Check sheet for the drawn part. Datum: minimum x, y, z corner. Units: mm. A direction names the side the tool comes from. Coordinates: 2 decimals unless noted, no trailing zeros. Loops run counter-clockwise (first coordinate to the right, second up) from the corner with the lowest first, then second, coordinate; pieces in that order, holes last.
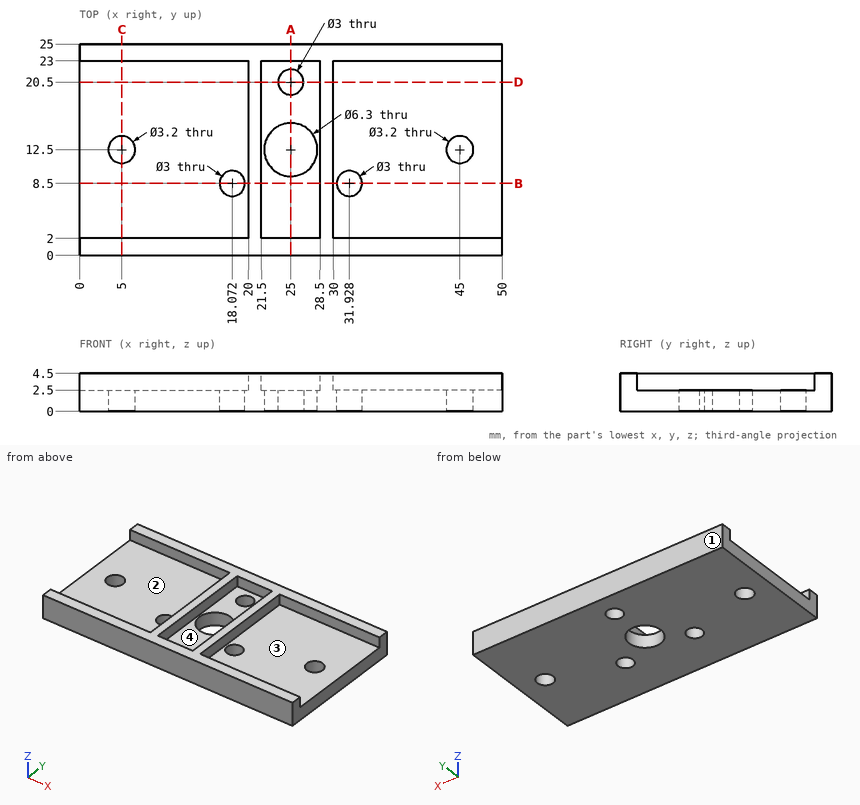
1) Section check C-C on x = 5. Enter the section's corners in (y, z), plus the area to 3 significant figures.
Answer sheet:
outline: (0, 0) - (10.9, 0) - (10.9, 2.5) - (2, 2.5) - (2, 4.5) - (0, 4.5) - close; (14.1, 0) - (25, 0) - (25, 4.5) - (23, 4.5) - (23, 2.5) - (14.1, 2.5) - close
area: 62.5 mm2
2) Mould release check, pull along X, two halves, no side actions. Record for the marked faces 3 and 4: +X half, -X half, draft (parallel to the pull), parting line (faces both ways), or undercut.
Answer sheet:
face 3: draft
face 4: undercut
3) Section check D-D on y = 20.5. Enter the section's corners in (x, z), plus the area to 4 significant figures.
Answer sheet:
outline: (0, 0) - (23.5, 0) - (23.5, 2.5) - (21.5, 2.5) - (21.5, 4.5) - (20, 4.5) - (20, 2.5) - (0, 2.5) - close; (26.5, 0) - (50, 0) - (50, 2.5) - (30, 2.5) - (30, 4.5) - (28.5, 4.5) - (28.5, 2.5) - (26.5, 2.5) - close
area: 123.5 mm2
4) Scan lines: line 1 (Y direction, x = 25, z = 1.2); line 2 (X direction, y = 8.5, z = 1.8); line 3 (X direction, y = 3, z = 2.55). Record each from-to range of solid material in increasing order.
Answer sheet:
line 1: y = 0 to 9.35, 15.65 to 19, 22 to 25
line 2: x = 0 to 16.57, 19.57 to 30.43, 33.43 to 50
line 3: x = 20 to 21.5, 28.5 to 30
5) Depth check by flat-ended pin: pin 1 (1 mm diameter, centred on x = 17.5, y = 3, fed in from +Z); pin 2 (2.5 mm diameter, centred on x = 45, y = 12.5, fed in from +Z); pin 3 (1.6 mm diameter, centred on y = 17.5, z = 4, fed in from +X); pin 4 (1.6 mm diameter, centred on y = 10.5, z = 3.5, fed in from -X). Enter the tip coordinate at first touch or a pass-through.
Answer sheet:
pin 1: stops at z = 2.5
pin 2: passes through
pin 3: stops at x = 30
pin 4: stops at x = 20
6) Section check A-A on x = 25. Enter the section's corners in (y, z).
Answer sheet:
outline: (0, 0) - (9.35, 0) - (9.35, 2.5) - (2, 2.5) - (2, 4.5) - (0, 4.5) - close; (15.65, 0) - (19, 0) - (19, 2.5) - (15.65, 2.5) - close; (22, 0) - (25, 0) - (25, 4.5) - (23, 4.5) - (23, 2.5) - (22, 2.5) - close
7) Section check B-B on y = 8.5. Enter the section's corners in (x, z).
Answer sheet:
outline: (0, 0) - (16.57, 0) - (16.57, 2.5) - (0, 2.5) - close; (19.57, 0) - (30.43, 0) - (30.43, 2.5) - (30, 2.5) - (30, 4.5) - (28.5, 4.5) - (28.5, 2.5) - (21.5, 2.5) - (21.5, 4.5) - (20, 4.5) - (20, 2.5) - (19.57, 2.5) - close; (33.43, 0) - (50, 0) - (50, 2.5) - (33.43, 2.5) - close
8) Set-up check for the marked faces 1 and 2: record each of +Z, -Z, +X, -X, +Y, -Y from which the full face is reachable in a straight line by a thin tool's end or side.
Answer sheet:
face 1: +Z, -Z, +X, -X, +Y
face 2: +Z, -X
